Here's how the part is built. I have some questions about the finished solid (model axes, mm). A direction names the side the tool comes from. Give positions to 0.01 mm unless a question says otherwise; leave off trailing zeros. Loops run counter-clockwise (first coordinate to the right, second up) from the corner with the lowest first, then second, coordinate; pieces in that order, holes last. Notation, with made-up numbers: (35, 45) - (81, 45) arc R6 ccw to (81, 53) - close; hole circle Ø1 at (-27.75, 0.25). An arc over 180 degrees is marked (long way). Return JSON: item names as keys, results as strings. Group by question number.
(1) For P1, Ø7, axis at y = 30, z = 0.5, coming from the +X side; P2, Ø4, axis at y = 15, z = 0, coming from the -X side; P3, Ø6.5, axis at x = 35, z = 0, coming from the +Y side, each with a flat end and sliding along its axis, tell me the tip position at first contact or that it passes through.
(2) If we mould it in two halves opening along X, with no side actions, what happens to faces 1 (the flat face through (0, 22, 0)), 2 (the cylindrical face through (40, 1, -4.9)), 3 (the cylindrical face through (17.26, 0.38, 1.18))? For each: released by +X, released by -X, zero draft, split by the parting line, or undercut.
(3) I need wall thicknesses on probe 1 along Z at (x, y) = (15, 0.25); probe 2 along Y at (x, z) = (28.5, 5.25). Which ranges of each line are inside material? Lowest first, please. Write a range as [from, to].
(4) If we section it at C-C (y = 10.5): Please give me the cut outline in (x, z).
(5) If we section it at A-A (x = 15): Please give me the cut outline in (y, z).
(6) On a 3-axis mill with a long thin cutter (end or side, diameter ignored), from which of +Z, -Z, +X, -X, +Y, -Y can I reach the whole of each face in a straight line? I mean faces 4 (the flat face through (22, 2, 0)), 5 (the flat face through (23, 0, 0)). Say none if no direction works.
```python
from build123d import *

# Parameters (mm, degrees)
BOSS_EXTRU_1_DEPTH                         = 7
CONG_1_R                                   = 7
FRAISAGE_POUR_VIS_T_TE_FRAIS_E_6_2_COUNT   = 2
FRAISAGE_POUR_VIS_T_TE_FRAIS_E_6_2_PITCH   = 20
FRAISAGE_POUR_VIS_T_TE_FRAIS_E_6_3_A_COUNT = 2
FRAISAGE_POUR_VIS_T_TE_FRAIS_E_6_3_A_PITCH = 20


with BuildPart() as part:
    # Esquisse1 → Boss.-Extru.1 (new, symmetric)
    with BuildSketch(Plane.XY):
        with BuildLine():
            Line((0, 3), (0, 42))
            Line((0, 42), (2, 42))
            Line((2, 42), (2, 3))
            ThreePointArc((2, 3), (2.292893219, 2.292893219), (3, 2))
            Line((3, 2), (42, 2))
            Line((42, 2), (42, 0))
            Line((42, 0), (3, 0))
            ThreePointArc((3, 0), (0.878679656, 0.878679656), (0, 3))
        make_face()
    extrude(amount=BOSS_EXTRU_1_DEPTH, both=True)

    # Congé1
    cong_1_edges = [part.edges().sort_by_distance(p)[0] for p in [
        (1, 42, -7),
        (1, 42, 7),
        (42, 1, -7),
        (42, 1, 7),
    ]]
    fillet(cong_1_edges, radius=CONG_1_R - 0.0001)  # a hair under: the kernel refuses the full size

    # Esquisse2 → Fraisage pour vis _ t_te frais_e _ 6 pan (revolve, cut)
    with BuildSketch(Plane(origin=(35, 2, 0), x_dir=(0, 0, 1), z_dir=(1, 0, 0))):
        Polygon((0, 0), (0, 2), (2.55, 2), (2.55, 1.25), (3.8, 0), align=None)
    fraisage_pour_vis_t_te_frais_e_6_pan = revolve(axis=Axis((35, 8.35, 0), (0, -1, 0)), mode=Mode.SUBTRACT)

    # Fraisage pour vis _ t_te frais_e _ 6 2: Fraisage pour vis _ t_te frais_e _ 6 pan ×2
    with Locations(*[(-i * FRAISAGE_POUR_VIS_T_TE_FRAIS_E_6_2_PITCH, 0, 0) for i in range(1, FRAISAGE_POUR_VIS_T_TE_FRAIS_E_6_2_COUNT)]):
        add(fraisage_pour_vis_t_te_frais_e_6_pan, mode=Mode.SUBTRACT)

    # Esquisse4 → Fraisage pour vis _ t_te frais_e _ 6 3 (revolve, cut)
    with BuildSketch(Plane(origin=(2, 35, 0), x_dir=(0, 0, -1), z_dir=(0, 1, 0))):
        Polygon((0, 0), (0, 2), (2.55, 2), (2.55, 1.25), (3.8, 0), align=None)
    fraisage_pour_vis_t_te_frais_e_6_3 = revolve(axis=Axis((8.35, 35, 0), (-1, 0, 0)), mode=Mode.SUBTRACT)

    # Fraisage pour vis _ t_te frais_e _ 6 3 a: Fraisage pour vis _ t_te frais_e _ 6 3 ×2
    with Locations(*[(0, -i * FRAISAGE_POUR_VIS_T_TE_FRAIS_E_6_3_A_PITCH, 0) for i in range(1, FRAISAGE_POUR_VIS_T_TE_FRAIS_E_6_3_A_COUNT)]):
        add(fraisage_pour_vis_t_te_frais_e_6_3, mode=Mode.SUBTRACT)


solid = part.part
```
Values:
{
 "1": {"P1": "x = 2", "P2": "through", "P3": "y = 1.45"},
 "2": {"face 1": "released by -X", "face 2": "released by +X", "face 3": "undercut"},
 "3": {"probe 1": "[-7, -2.55], [2.55, 7]", "probe 2": "[0, 2]"},
 "4": {"outline": "(0, -7) - (2, -7) - (2, 7) - (0, 7) - close"},
 "5": {"outline": "(0, -7) - (2, -7) - (2, -3.8) - (0.75, -2.55) - (0, -2.55) - close; (0, 2.55) - (0.75, 2.55) - (2, 3.8) - (2, 7) - (0, 7) - close"},
 "6": {"face 4": "+Z, -Z, +X, +Y", "face 5": "+Z, -Z, +X, -X, -Y"}
}
